from build123d import *

# Parameters (mm, degrees)
F0_W     = 115.9510612488
F0_H     = 232.1095168591
F1_DEPTH = 25.4
F2_DEPTH = 50.8
F0_W_2   = 8.6233839393
F0_H_2   = 51.5415742993
F0_W_3   = 10.8864195645
F0_H_3   = 76.7579004169
F0_W_4   = 10.6456745416
F0_H_4   = 91.7214006186
F0_R     = 21.2419727644
F0_W_5   = 34.5992818475
F0_H_5   = 30.4277390242
F3_DEPTH = 25.4
F4_DEPTH = 43.18
F5_DEPTH = 22.86
F6_R     = 9.647506056
F6_R_2   = 5.7913302068
F7_DEPTH = 25.4


with BuildPart() as f1:
    # F0 (on Top) → F1 (new body)
    with BuildSketch(Plane.XY):
        Polygon((-242.6905930042, -183.078199625), (0, -183.078199625), (242.6905930042, -183.078199625), (242.6905930042, 183.078199625), (-242.6905930042, 183.078199625), align=None)
        with Locations((-128.7101954222, 0)):
            Rectangle(F0_W, F0_H, mode=Mode.SUBTRACT)
        with BuildLine():
            ThreePointArc((-8.3529502331, -63.9360985563), (-42.5382359375, 48.4571455981), (64.479426767, 0))
            ThreePointArc((64.479426767, 0), (42.5382359375, -48.4571455981), (-8.3529502331, -63.9360985563))
        make_face(mode=Mode.SUBTRACT)
        with Locations((128.7101954222, 0)):
            Rectangle(F0_W, F0_H, mode=Mode.SUBTRACT)
    extrude(amount=F1_DEPTH)

    # F0 (on Top) → F2 (join)
    with BuildSketch(Plane.XY):
        with BuildLine():
            ThreePointArc((-8.3529502331, -63.9360985563), (42.5382359375, -48.4571455981), (64.479426767, 0))
            ThreePointArc((64.479426767, 0), (-42.5382359375, 48.4571455981), (-8.3529502331, -63.9360985563))
        make_face()
        with BuildLine():
            ThreePointArc((0, 60.5718467831), (42.8307636094, 42.8307636094), (60.5718467831, 0))
            ThreePointArc((60.5718467831, 0), (42.8307636094, -42.8307636094), (0, -60.5718467831))
            ThreePointArc((0, -60.5718467831), (-60.5718467831, 0), (0, 60.5718467831))
        make_face(mode=Mode.SUBTRACT)
    extrude(amount=F2_DEPTH)

    # F0 (on Top) → F3 (join)
    with BuildSketch(Plane.XY):
        with BuildLine():
            Line((0, -60.5718467831), (0, 60.5718467831))
            ThreePointArc((0, 60.5718467831), (-60.5718467831, 0), (0, -60.5718467831))
        make_face()
        with Locations((-46.3319979608, 0)):
            Rectangle(F0_W_2, F0_H_2, mode=Mode.SUBTRACT)
        with Locations((-30.0273634493, 0)):
            Rectangle(F0_W_3, F0_H_3, mode=Mode.SUBTRACT)
        with Locations((-12.9544232041, 0)):
            Rectangle(F0_W_4, F0_H_4, mode=Mode.SUBTRACT)
        with BuildLine():
            ThreePointArc((0, -60.5718467831), (42.8307636094, -42.8307636094), (60.5718467831, 0))
            ThreePointArc((60.5718467831, 0), (42.8307636094, 42.8307636094), (0, 60.5718467831))
            Line((0, 60.5718467831), (0, -60.5718467831))
        make_face()
        with Locations((25.1728594303, -21.464029327)):
            Circle(F0_R, mode=Mode.SUBTRACT)
        with Locations((20.2057100832, 26.9539654255)):
            Rectangle(F0_W_5, F0_H_5, mode=Mode.SUBTRACT)
    extrude(amount=F3_DEPTH)

    # F0 (on Top) → F4 (join)
    with BuildSketch(Plane.XY):
        with Locations((-46.3319979608, 0)):
            Rectangle(F0_W_2, F0_H_2)
        with Locations((-30.0273634493, 0)):
            Rectangle(F0_W_3, F0_H_3)
        with Locations((-12.9544232041, 0)):
            Rectangle(F0_W_4, F0_H_4)
    extrude(amount=F4_DEPTH)

    # F0 (on Top) → F5 (join)
    with BuildSketch(Plane.XY):
        with Locations((-128.7101954222, 0)):
            Rectangle(F0_W, F0_H)
        with Locations((20.2057100832, 26.9539654255)):
            Rectangle(F0_W_5, F0_H_5)
        with Locations((25.1728594303, -21.464029327)):
            Circle(F0_R)
        with Locations((128.7101954222, 0)):
            Rectangle(F0_W, F0_H)
    extrude(amount=F5_DEPTH)

    # F6 (on face) → F7 (join)
    with BuildSketch(Plane.XY.offset(25.4)):
        with Locations((-216.0538285971, 0)):
            Circle(F6_R)
        with Locations((-35.002566874, -116.0547584295)):
            Circle(F6_R_2)
        with BuildLine():
            Line((0, 102.9595498758), (0, 119.0302903933))
            ThreePointArc((0, 119.0302903933), (-8.0353702587, 110.9949201345), (0, 102.9595498758))
        make_face()
        with BuildLine():
            ThreePointArc((0, 102.9595498758), (5.6818647993, 105.3130553353), (8.0353702587, 110.9949201345))
            ThreePointArc((8.0353702587, 110.9949201345), (5.6818647993, 116.6767849338), (0, 119.0302903933))
            Line((0, 119.0302903933), (0, 102.9595498758))
        make_face()
        with Locations((216.0538285971, 0)):
            Circle(F6_R)
    extrude(amount=F7_DEPTH)


solid = f1.part
Source: CAD feature listing. Evaluate the final solid. Frame: model axes, mm. A direction names the side the tool comes from. Coordinates: 2 decimals unless noted, no trailing zeros. Loops run counter-clockwise (first coordinate to the right, second up) from the corner with the lowest first, then second, coordinate; pieces in that order, holes last. Notation, with made-up numbers: (23, 71.5) -> (41, 71.5) arc R21 cw to (41, 93.5) -> close; hole circle Ø6 at (-27, 57). An arc over 180 degrees is marked (long way). Answer in a Markdown table with one row per item. Add a question column.
Q1. Ray query, line 1 along X through (y, z) = (20, 36); line 2 along Z through (x, y) = (168.5, -116.5); line 3 along X through (y, z) = (-6, 43.5). Return the intervals inside material, ascending.
Q2. Contact query for flat-ended pins moving along their axis: pin 1 Ø5.5 at (y, z) = (-13.5, 31) entering from -X; pin 2 Ø9 at (y, z) = (8.5, 35.5) entering from -X; pin 3 Ø8 at (y, z) = (6.5, 40) entering from -X; pin 4 Ø5 at (x, y) = (-37.5, -52.5) entering from -Z. Output: stop coordinate, or through.
Q3. Section B-B on x = 174. Return the cut outline in (y, z).
Q4. Pull-direction query (X, two-part tool) for faces 1 (the face through (-3, -183.078, 13)), 2 (the face through (-13, 45.861, 34)); classes: pulls with the +X half, pulls with the -X half, needs draft (parallel to the pull), parting line crosses it, or undercut.
Q5. Section C-C on y = 140. Return the cut outline in (x, z), and give its area (3 significant figures).
Q6. Reachability of faces 3 (the face through (-57, 43, 25.4)), 4 (the face through (-3, 3, 0)) from +Z, -Z, +X, -X, +Y, -Y: full face, straight path, thin tool, end or side. Return the list, or none.
Q7. Section A-A on y = 96. Return the cut outline in (x, z).
Computed values:
| question | item | result |
|---|---|---|
| 1 | line 1 | x = -61.3 to -57.17, -50.64 to -42.02, -35.47 to -24.58, -18.28 to -7.63, 57.17 to 61.3 |
| 1 | line 2 | z = 0 to 25.4 |
| 1 | line 3 | x = -223.61 to -208.5, -64.2 to -60.27, 60.27 to 64.2, 208.5 to 223.61 |
| 2 | pin 1 | stops at x = -63.58 |
| 2 | pin 2 | stops at x = -224.83 |
| 2 | pin 3 | stops at x = -225.37 |
| 2 | pin 4 | stops at z = 0 |
| 3 | outline | (-183.08, 0) -> (183.08, 0) -> (183.08, 25.4) -> (116.05, 25.4) -> (116.05, 22.86) -> (-116.05, 22.86) -> (-116.05, 25.4) -> (-183.08, 25.4) -> close |
| 4 | face 1 | needs draft |
| 4 | face 2 | undercut |
| 5 | outline | (-242.69, 0) -> (242.69, 0) -> (242.69, 25.4) -> (-242.69, 25.4) -> close |
| 5 | area | 12,300 mm^2 |
| 6 | face 3 | +Z |
| 6 | face 4 | -Z, +X, -X, +Y, -Y |
| 7 | outline | (-242.69, 0) -> (242.69, 0) -> (242.69, 25.4) -> (186.69, 25.4) -> (186.69, 22.86) -> (70.73, 22.86) -> (70.73, 25.4) -> (-70.73, 25.4) -> (-70.73, 22.86) -> (-186.69, 22.86) -> (-186.69, 25.4) -> (-242.69, 25.4) -> close |
